Could you check a few things on this drawing? It's one solid part, dimensions in mm from its lowest x, y, z. Give positions to 0.01 mm unless a question says otherwise; leave off trailing zeros. Write each loop counter-clockwise with the first axis right and the second up, starting at its lowest first coordinate (ties: lowest second). Pieces come first, ordered by that corner, then holes. Notation, with made-up numbers: (-11.5, 60.5) -> (12.5, 60.5) arc R24 cw to (12.5, 85.5) -> close; hole circle Ø8 at (-39, 24.5). An arc over 180 degrees is marked (long way). Answer as CSV lines item,"result". Start each with the question number.
1. If we section it at B-B on x = 41: Write out the boundary of the cut face in (y, z).
2. I'm going to push flat-ended pins straight in: P1, Ø0.6, axis at x = 70.5, z = 0.5, coming from the -Y side; P2, Ø12, axis at x = 50, y = 29.5, coming from the -Z side; P3, Ø0.6, axis at x = 0.5, z = 0.5, coming from the -Y side. Where does each tip first touch, or does it pass through?
3. I need wall thicknesses on line 1 (X direction, y = 13, z = 1.1); line 2 (Y direction, x = 37, z = 1.1); line 3 (X direction, y = 8.5, z = 0.9). Which ranges of each line are inside material? Lowest first, please. Write a range as [from, to].
4. If we section it at D-D on y = 26: Write out the boundary of the cut face in (x, z), plus the area to 3 significant figures.
5. If we section it at C-C on y = 15: Write out the boundary of the cut face in (x, z), plus the area to 3 significant figures.
6. If we section it at A-A on z = 0.25: Count the separate pieces of the cut face and the enclosed holes in it, plus the area to 3 significant figures.
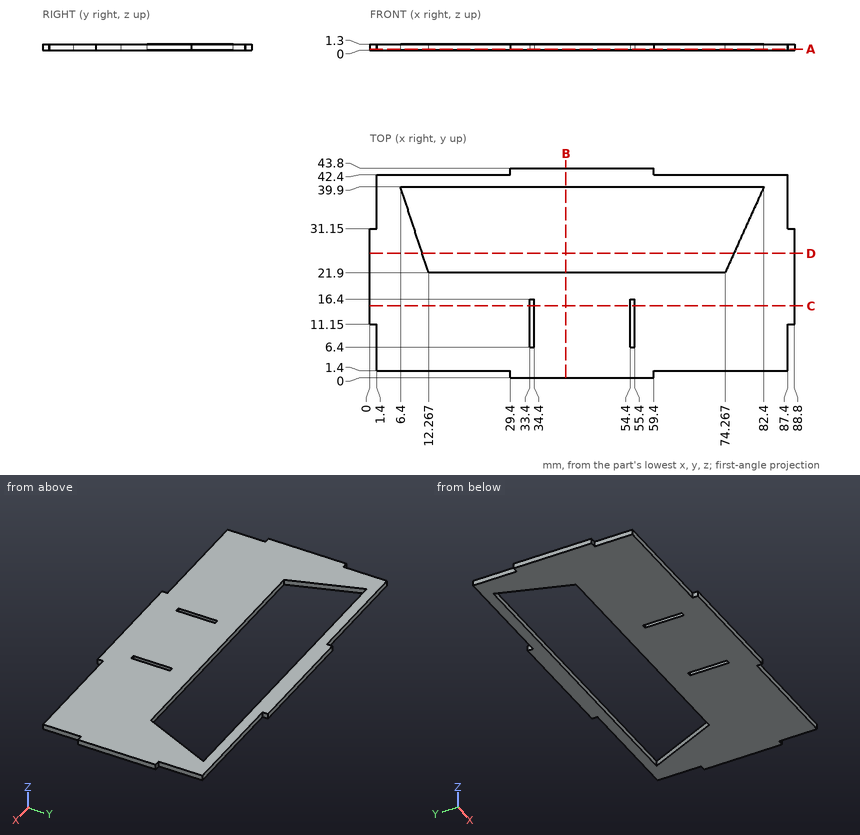
Computed values:
1,outline,"(0, 0) -> (21.9, 0) -> (21.9, 1.3) -> (0, 1.3) -> close; (39.9, 0) -> (43.8, 0) -> (43.8, 1.3) -> (39.9, 1.3) -> close"
2,P1,"stops at y = 1.4"
2,P2,"passes through"
2,P3,"stops at y = 11.15"
3,line 1,"x = [0, 33.4], [34.4, 54.4], [55.4, 88.8]"
3,line 2,"y = [0, 21.9], [39.9, 43.8]"
3,line 3,"x = [1.4, 33.4], [34.4, 54.4], [55.4, 87.4]"
4,outline,"(0, 0) -> (10.93, 0) -> (10.93, 1.3) -> (0, 1.3) -> close; (76.12, 0) -> (88.8, 0) -> (88.8, 1.3) -> (76.12, 1.3) -> close"
4,area,"30.7 mm2"
5,outline,"(0, 0) -> (33.4, 0) -> (33.4, 1.3) -> (0, 1.3) -> close; (34.4, 0) -> (54.4, 0) -> (54.4, 1.3) -> (34.4, 1.3) -> close; (55.4, 0) -> (88.8, 0) -> (88.8, 1.3) -> (55.4, 1.3) -> close"
5,area,"113 mm2"
6,separate pieces,"1"
6,enclosed holes,"3"
6,area,"2,400 mm2"
